```python
from build123d import *

# Parameters (mm, degrees)
SKETCH1_R               = 6.35
BASIC_ROD_DEPTH         = 10.7696
BASIC_ROD_DEPTH_BACK    = 10.7696
THEX_DEPTH              = 10.7696
SKETCH2_R               = 2.9972
INTERNAL_CUT_DEPTH      = 14.3096
INTERNAL_CUT_DEPTH_BACK = 14.3096


with BuildPart() as part:
    # Sketch1 → Basic Rod (new body, two sides)
    with BuildSketch(Plane.XY) as basic_rod_sk:
        Circle(SKETCH1_R)
    extrude(amount=BASIC_ROD_DEPTH)
    extrude(basic_rod_sk.sketch, amount=-BASIC_ROD_DEPTH_BACK)

    # Sketch8 → THex (add, symmetric)
    with BuildSketch(Plane.XY):
        with BuildLine():
            Line((-0.888411378, 6.819423871), (-5.461588622, 4.179098758))
            ThreePointArc((-5.461588622, 4.179098758), (-5.955700003, 3.438525), (-6.35, 2.640325113))
            Line((-6.35, 2.640325113), (-6.35, -2.640325113))
            ThreePointArc((-6.35, -2.640325113), (-5.955700003, -3.438525), (-5.461588622, -4.179098758))
            Line((-5.461588622, -4.179098758), (-0.888411378, -6.819423871))
            ThreePointArc((-0.888411378, -6.819423871), (0, -6.87705), (0.888411378, -6.819423871))
            Line((0.888411378, -6.819423871), (5.461588622, -4.179098758))
            ThreePointArc((5.461588622, -4.179098758), (5.955700003, -3.438525), (6.35, -2.640325113))
            Line((6.35, -2.640325113), (6.35, 2.640325113))
            ThreePointArc((6.35, 2.640325113), (5.955700003, 3.438525), (5.461588622, 4.179098758))
            Line((5.461588622, 4.179098758), (0.888411378, 6.819423871))
            ThreePointArc((0.888411378, 6.819423871), (0, 6.87705), (-0.888411378, 6.819423871))
        make_face()
    extrude(amount=THEX_DEPTH, both=True)

    # Sketch7 → 1stSnapRing (revolve)
    with BuildSketch(Plane(origin=(0, 0, 0), x_dir=(0, 0, -1), z_dir=(1, 0, 0))):
        Polygon((-10.7696, 5.9436), (-11.7856, 5.9436), (-11.7856, 6.35), (-12.8016, 6.35), (-13.3096, 5.842), (-13.3096, 0), (-10.7696, 0), align=None)
    f_1stsnapring = revolve(axis=Axis((0, 0, -38.2778), (0, 0, 1)))

    # 2ndSnapRing: 1stSnapRing across plane
    add(f_1stsnapring.mirror(Plane.XY))

    # Sketch2 → Internal Cut (cut, two sides)
    with BuildSketch(Plane.XY) as internal_cut_sk:
        Circle(SKETCH2_R)
    extrude(amount=INTERNAL_CUT_DEPTH, mode=Mode.SUBTRACT)
    extrude(internal_cut_sk.sketch, amount=-INTERNAL_CUT_DEPTH_BACK, mode=Mode.SUBTRACT)


solid = part.part
```
The model under review builds one solid part; all positions refer to its coordinate system, in mm. A direction names the side the tool comes from. Coordinates: 2 decimals unless noted, no trailing zeros. Write each loop counter-clockwise with the first axis right and the second up, starting at its lowest first coordinate (ties: lowest second). Pieces come first, ordered by that corner, then holes. Notation, with made-up numbers: (-24.75, 77) -> (15.25, 77) arc R24 cw to (15.25, 92) -> close; hole circle Ø2 at (28, -29). An arc over 180 degrees is marked (long way). One line per item, written item: value. Start each with the question number.
Q1. For faces 4 (the face through (-1.785, 5.669, -11.285)), 5 (the face through (6.2, -1.38, 12.3)), 6 (the face through (6.2, -1.38, -12.3)), list the 3-axis set-ups (+Z, -Z, +X, -X, +Y, -Y) from which the entire face can be reached by the end or side of a thin tool; tool diameter is ignored.
Q2. To check wall thickness, follow probe 1 along X at (y, z) = (0, 1.5); probe 2 along Y at (x, z) = (0, -2); probe 3 along Z at (x, y) = (1, 6). State the ranges of each line that lie inside material, in increasing order.
Q3. Add section A-A, the plane x = 0. Give the boundary of the cut face in (y, z), then the cut area to 3 significant figures.
Q4. Add section C-C, the plane z = 3. Give the boundary of the cut face in (x, y), then the cut area to 3 significant figures.
Q5. Clearance check with flat-ended pins moving along their axes: P1, Ø6.5, axis at x = 0.5, y = 0, coming from the -Z side; P2, Ø1.5, axis at y = -4.5, z = -9.5, coming from the +X side; P3, Ø1.5, axis at x = -4, z = 1.5, coming from the -Y side. State where each tip first meets the part, or that it passes through.
Q6. Add section B-B, the plane y = 0. Give the boundary of the cut face in (x, z).
Q7. The part is to be moulded in two halves that separate along Z. For faces 1 (the face through (-1, -3, 13.31)), 2 (the face through (0.012, 6.877, 0.151)), 3 (the face through (-1.785, 5.669, 11.285)), say which applies: +Z half, -Z half, draft (parallel to the pull), parting line (faces both ways), or undercut.
Response:
1. face 4: none
1. face 5: +Z
1. face 6: -Z
2. probe 1: -6.35 to -3, 3 to 6.35
2. probe 2: -6.88 to -3, 3 to 6.88
2. probe 3: -13.07 to -11.79, -10.77 to 10.77, 11.79 to 13.07
3. outline: (-6.88, -10.77) -> (-5.94, -10.77) -> (-5.94, -11.79) -> (-6.35, -11.79) -> (-6.35, -12.8) -> (-5.84, -13.31) -> (-3, -13.31) -> (-3, 13.31) -> (-5.84, 13.31) -> (-6.35, 12.8) -> (-6.35, 11.79) -> (-5.94, 11.79) -> (-5.94, 10.77) -> (-6.88, 10.77) -> close; (3, -13.31) -> (5.84, -13.31) -> (6.35, -12.8) -> (6.35, -11.79) -> (5.94, -11.79) -> (5.94, -10.77) -> (6.88, -10.77) -> (6.88, 10.77) -> (5.94, 10.77) -> (5.94, 11.79) -> (6.35, 11.79) -> (6.35, 12.8) -> (5.84, 13.31) -> (3, 13.31) -> close
3. area: 199 mm²
4. outline: (-6.35, -2.64) arc R6.88 ccw to (-5.46, -4.18) -> (-0.89, -6.82) arc R6.88 ccw to (0.89, -6.82) -> (5.46, -4.18) arc R6.88 ccw to (6.35, -2.64) -> (6.35, 2.64) arc R6.88 ccw to (5.46, 4.18) -> (0.89, 6.82) arc R6.88 ccw to (-0.89, 6.82) -> (-5.46, 4.18) arc R6.88 ccw to (-6.35, 2.64) -> close; hole circle Ø5.99 at (0, 0)
4. area: 109 mm²
5. P1: z = -13.31
5. P2: x = 5.76
5. P3: y = -5.46
6. outline: (-6.35, -12.8) -> (-5.84, -13.31) -> (-3, -13.31) -> (-3, 13.31) -> (-5.84, 13.31) -> (-6.35, 12.8) -> (-6.35, 11.79) -> (-5.94, 11.79) -> (-5.94, 10.77) -> (-6.35, 10.77) -> (-6.35, -10.77) -> (-5.94, -10.77) -> (-5.94, -11.79) -> (-6.35, -11.79) -> close; (3, -13.31) -> (5.84, -13.31) -> (6.35, -12.8) -> (6.35, -11.79) -> (5.94, -11.79) -> (5.94, -10.77) -> (6.35, -10.77) -> (6.35, 10.77) -> (5.94, 10.77) -> (5.94, 11.79) -> (6.35, 11.79) -> (6.35, 12.8) -> (5.84, 13.31) -> (3, 13.31) -> close
7. face 1: +Z half
7. face 2: draft
7. face 3: undercut
